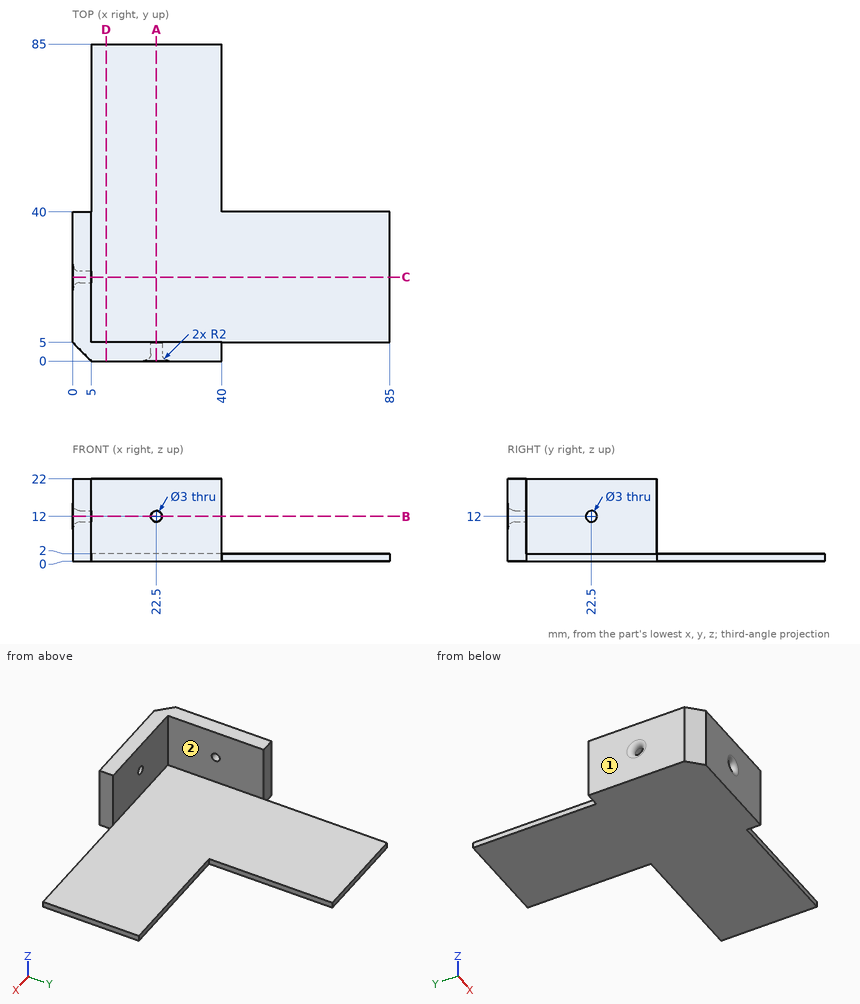
The figure shows three views and two pictorial views of one solid part (mm, origin at its lowest corner). Answer the questions. A direction names the side the tool comes from. Round coordinates to 2 decimals unless told otherwise and drop trailing zeros. Write each loop counter-clockwise with the first axis right and the second up, starting at its lowest first coordinate (ties: lowest second). Pieces come first, ordered by that corner, then holes. Notation, with made-up numbers: (84, -28) -> (117, -28) arc R32 ccw to (117, 6) -> close; hole circle Ø2 at (77.25, -25). An arc over 180 degrees is marked (long way). Write each question's results on one line, items separated by ' | '.
Q1. Section A-A, the plane x = 22.5 is taken. Write down the section's boundary in (y, z).
Data:
outline: (0, 0) -> (85, 0) -> (85, 2) -> (5, 2) -> (5, 10.5) -> (2, 10.5) arc R2 ccw to (0, 8.5) -> close; (0, 15.5) arc R2 ccw to (2, 13.5) -> (5, 13.5) -> (5, 22) -> (0, 22) -> close
Q2. Straight lines are drawn through the part: line 1 along X through (y, z) = (3, 12); line 2 along Z through (x, y) = (22.5, 2.9); line 3 along Y through (x, z) = (35, 8.75). For each, find the intervals that lie inside material, in ascending order. Write a range as [from, to].
Data:
line 1: [2, 21], [24, 40] | line 2: [0, 10.5], [13.5, 22] | line 3: [0, 5]
Q3. Which of the six approach directions +Z, -Z, +X, -X, +Y, -Y give full straight-line access (tool end or side, diameter ignored) to the marked faces 1 and 2?
Data:
face 1: +Z, -Z, -X, +Y, -Y | face 2: +Z, +X, +Y
Q4. Section B-B, the plane z = 12 is taken. Write down the section's boundary in (x, y).
Data:
outline: (0, 5) -> (5, 0) -> (19, 0) arc R2 ccw to (21, 2) -> (21, 5) -> (5, 5) -> (5, 21) -> (2, 21) arc R2 ccw to (0, 19) -> close; (0, 26) arc R2 ccw to (2, 24) -> (5, 24) -> (5, 40) -> (0, 40) -> close; (24, 2) arc R2 ccw to (26, 0) -> (40, 0) -> (40, 5) -> (24, 5) -> close
Q5. Flat-ended cylindrical pins translate along their axes: P1, Ø2.5, axis at y = 2.5, z = 15, coming from the +X side; P2, Ø2.5, axis at y = 22.5, z = 12, coming from the +X side; P3, Ø1.6, axis at x = 63, z = 1.5, coming from the +Y side; P4, Ø1.6, axis at x = 67, z = 1.5, coming from the -Y side. Find the tip coordinate at first contact, or state that the pin passes through.
Data:
P1: x = 40 | P2: through | P3: y = 40 | P4: y = 5
Q6. Section D-D, the plane x = 9 is taken. Write down the section's boundary in (y, z).
Data:
outline: (0, 0) -> (85, 0) -> (85, 2) -> (5, 2) -> (5, 22) -> (0, 22) -> close
